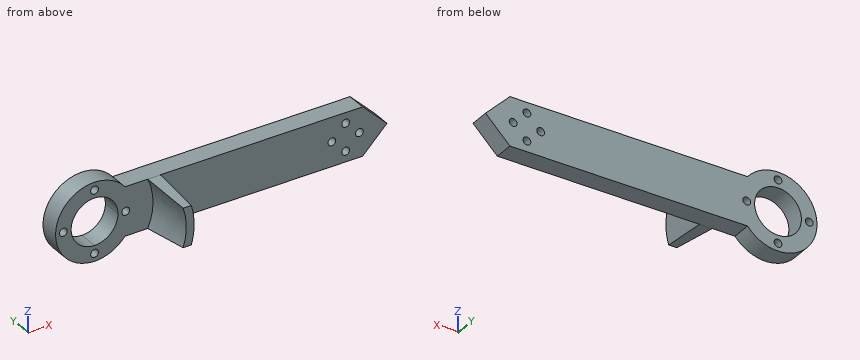
```python
from build123d import *

# Parameters (mm, degrees)
SKETCH_1_R          = 2
EXTRUDE_1_DEPTH     = 10
SKETCH_2_R          = 2
CUT_EXTRUDE_1_DEPTH = 10


with BuildPart() as part:
    # 스케치1 → 보스-돌출1 (new body)
    with BuildSketch(Plane(origin=(0, 0, 0), x_dir=(1, 0, 0), z_dir=(0, 1, 0))):
        with BuildLine():
            ThreePointArc((-59.387505004, 12.5), (-95, 0), (-59.387505004, -12.5))
            Line((-59.387505004, -12.5), (62.5, -12.5))
            Line((62.5, -12.5), (75, 0))
            Line((75, 0), (62.5, 12.5))
            Line((62.5, 12.5), (-59.387505004, 12.5))
        make_face()
        with Locations(Location((-75, -16, 0), (0, 0, 270))):
            Circle(SKETCH_1_R, mode=Mode.SUBTRACT)
        with Locations(Location((-91, 0, 0), (0, 0, 270))):
            Circle(SKETCH_1_R, mode=Mode.SUBTRACT)
        with BuildLine():
            ThreePointArc((-75, 12), (-66.514718626, 8.485281374), (-63, 0))
            ThreePointArc((-63, 0), (-83.485281374, -8.485281374), (-75, 12))
        make_face(mode=Mode.SUBTRACT)
        with BuildLine():
            ThreePointArc((-61, 0), (-59, 2), (-57, 0))
            ThreePointArc((-57, 0), (-59, -2), (-61, 0))
        make_face(mode=Mode.SUBTRACT)
        with Locations(Location((-75, 16, 0), (0, 0, 270))):
            Circle(SKETCH_1_R, mode=Mode.SUBTRACT)
    extrude(amount=EXTRUDE_1_DEPTH)

    # 스케치2 → 컷-돌출1 (cut)
    with BuildSketch(Plane(origin=(0, 0, 0), x_dir=(1, 0, 0), z_dir=(0, 1, 0))):
        with Locations(Location((53.786796564, 7.071067812, 0), (0, 0, 270))):
            Circle(SKETCH_2_R)
        with Locations(Location((60.857864376, 0, 0), (0, 0, 270))):
            Circle(SKETCH_2_R)
        with Locations(Location((46.715728753, 0, 0), (0, 0, 270))):
            Circle(SKETCH_2_R)
        with Locations(Location((53.786796564, -7.071067812, 0), (0, 0, 270))):
            Circle(SKETCH_2_R)
    extrude(amount=CUT_EXTRUDE_1_DEPTH, mode=Mode.SUBTRACT)

    # 스케치3 for 로프트1 → 로프트1 section 0
    with BuildSketch(Plane(origin=(0, 0, 0), x_dir=(1, 0, 0), z_dir=(0, 1, 0))):
        with BuildLine():
            Line((-41.239816351, 12.5), (-47.728219713, 12.5))
            # circular arc as an exact rational Bezier (weights 1, cos(half-angle), 1)
            Bezier((-47.728219713, 12.5), (-41.998854107, 0), (-47.728219713, -12.5), weights=[1, 0.909059343, 1])
            Line((-47.728219713, -12.5), (-41.239816351, -12.5))
            Bezier((-41.239816351, -12.5), (-36.611583234, 0), (-41.239816351, 12.5), weights=[1, 0.937782879, 1])
        make_face()
    # 스케치4 for 로프트1 → 로프트1 section 1
    with BuildSketch(Plane(origin=(0, -25, 0), x_dir=(1, 0, 0), z_dir=(0, 1, 0))):
        with BuildLine():
            Line((-45.657198498, -10), (-41.458980338, -10))
            Bezier((-41.458980338, -10), (-38.477556368, 0), (-41.458980338, 10), weights=[1, 0.958314847, 1])
            Line((-41.458980338, 10), (-45.657198498, 10))
            Bezier((-45.657198498, 10), (-42.249207615, 0), (-45.657198498, -10), weights=[1, 0.946541984, 1])
        make_face()
    loft()


solid = part.part
```
Geometry check sheet. Reference: the model listing, model coordinates, mm. Coordinates: 2 decimals unless noted, no trailing zeros. Loops run counter-clockwise (first coordinate to the right, second up) from the corner with the lowest first, then second, coordinate; pieces in that order, holes last.
Item 1: Sectioned sample at A-A, the plane z = 16. Record the boundary of the cut face in (x, y).
Item 2: Sectioned sample at B-B, the plane y = 1.5. Count the separate pieces of the cut face and the enclosed holes in it, then the cut area to 3 significant figures.
Item 3: Go/stop test with flat-tipped pins: pin 1 Ø5 at (x, y) = (25, 7) entering from +Z; pin 2 Ø3 at (x, z) = (-57.5, 6) entering from -Y; pin 3 Ø3 at (x, y) = (-1.5, 3) entering from -Z. Record where each tip stops, or that it passes through.
Item 4: Thickness scan on line 1 (X direction, y = 4.75, z = -16); line 2 (Y direction, x = -26.5, z = 7); line 3 (X direction, y = 1, z = 3.5). Record the ranges inside material, lowest first.
Item 5: Sectioned sample at C-C, the plane x = -19.5. Record the boundary of the cut face in (y, z), then the cut area to 3 significant figures.
Check result:
1. outline: (-87, 0) - (-77, 0) - (-77, 10) - (-87, 10) - close; (-73, 0) - (-63, 0) - (-63, 10) - (-73, 10) - close
2. separate pieces: 1
2. enclosed holes: 9
2. area: 3,830 mm2
3. pin 1: stops at z = 12.5
3. pin 2: stops at y = 0
3. pin 3: stops at z = -12.5
4. line 1: x = -87 to -77, -73 to -63
4. line 2: y = 0 to 10
4. line 3: x = -94.69 to -86.48, -63.52 to 71.5
5. outline: (0, -12.5) - (10, -12.5) - (10, 12.5) - (0, 12.5) - close
5. area: 250 mm2
